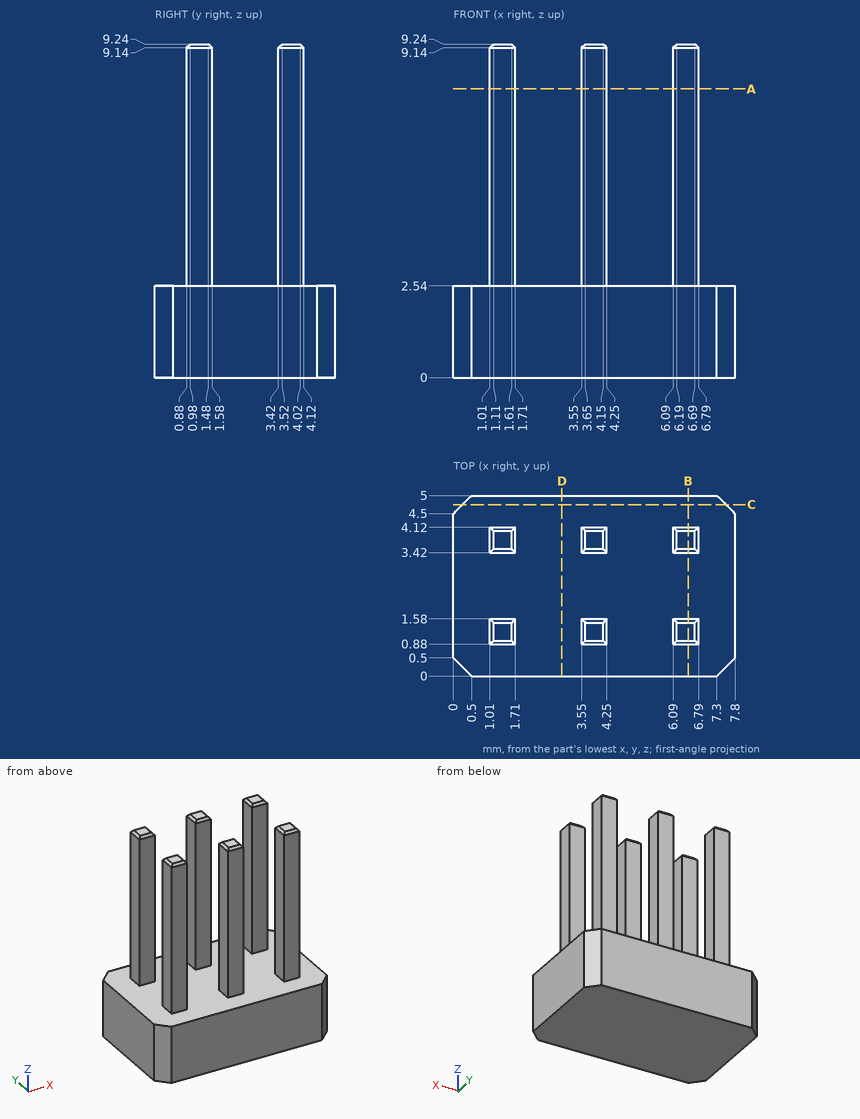
Can you work these out from the drawing? Everything is in mm from the part's minimum corner. Coordinates: 2 decimals unless noted, no trailing zeros. Write each loop counter-clockwise with the first axis right and the second up, starting at its lowest first coordinate (ties: lowest second). Pieces come first, ordered by that corner, then holes. Notation, with made-up numbers: (-0.75, -32.5) - (28.25, -32.5) arc R17 cw to (28.25, -22.5) - close; hole circle Ø6 at (-14.75, 86.5). An arc over 180 degrees is marked (long way). Use a Markdown table: item, result.
Q1. Please list where these lines run through material, in increasing order: L1, parallel to X at y = 1.1, z = 3; L2, parallel to Y at x = 4, z = 7.5.
Geometry check:
| item | result |
|---|---|
| L1 | x = 1.01 to 1.71, 3.55 to 4.25, 6.09 to 6.79 |
| L2 | y = 0.88 to 1.58, 3.42 to 4.12 |
Q2. Imagine slicing it at C-C (y = 4.75). List the corners of the cut face in (x, z) for me.
Geometry check:
| item | result |
|---|---|
| outline | (0.25, 0) - (7.55, 0) - (7.55, 2.54) - (0.25, 2.54) - close |
Q3. Imagine slicing it at B-B (x = 6.5). List the corners of the cut face in (y, z) for me.
Geometry check:
| item | result |
|---|---|
| outline | (0, 0) - (5, 0) - (5, 2.54) - (4.12, 2.54) - (4.12, 9.14) - (4.02, 9.24) - (3.52, 9.24) - (3.42, 9.14) - (3.42, 2.54) - (1.58, 2.54) - (1.58, 9.14) - (1.48, 9.24) - (0.98, 9.24) - (0.88, 9.14) - (0.88, 2.54) - (0, 2.54) - close |
Q4. Imagine slicing it at A-A (z = 8). List the corners of the cut face in (x, y) for me.
Geometry check:
| item | result |
|---|---|
| outline | (1.01, 0.88) - (1.71, 0.88) - (1.71, 1.58) - (1.01, 1.58) - close; (1.01, 3.42) - (1.71, 3.42) - (1.71, 4.12) - (1.01, 4.12) - close; (3.55, 0.88) - (4.25, 0.88) - (4.25, 1.58) - (3.55, 1.58) - close; (3.55, 3.42) - (4.25, 3.42) - (4.25, 4.12) - (3.55, 4.12) - close; (6.09, 0.88) - (6.79, 0.88) - (6.79, 1.58) - (6.09, 1.58) - close; (6.09, 3.42) - (6.79, 3.42) - (6.79, 4.12) - (6.09, 4.12) - close |
Q5. I'm going to push flat-ended pins straight in: pin 1 Ø2 at (x, z) = (5.5, 5.5) entering from -Y; pin 2 Ø0.8 at (y, z) = (1.5, 5) entering from +X; pin 3 Ø0.8 at (y, z) = (1, 5) entering from -X. Where does each tip first touch, or does it pass through?
Geometry check:
| item | result |
|---|---|
| pin 1 | stops at y = 0.88 |
| pin 2 | stops at x = 6.79 |
| pin 3 | stops at x = 1.01 |
Q6. Imagine slicing it at D-D (x = 3). List the corners of the cut face in (y, z) for me.
Geometry check:
| item | result |
|---|---|
| outline | (0, 0) - (5, 0) - (5, 2.54) - (0, 2.54) - close |
